Can you work these out from the model? Positions are in its coordinate system, mm. A direction names the side the tool comes from. Give positions to 0.01 mm unless a question says otherwise; leave off trailing zeros. Loops run counter-clockwise (first coordinate to the right, second up) from the corner with the lowest first, then second, coordinate; pieces in that order, holes last. Notation, with made-up numbers: (-3.75, 60) - (6.25, 60) arc R20 cw to (6.25, 99) - close; hole circle Ø11 at (49.5, -6.5). An arc over 180 degrees is marked (long way). Write item = value, one per line.
from build123d import *

# Parameters (mm, degrees)
BASE_DEPTH      = 10
ESQUISSE3_R     = 2.5
VIDE_TROU_DEPTH = 10
ESQUISSE4_R     = 4
AXE_DEPTH       = 90
CONG_5_R        = 1


with BuildPart() as part:
    # Esquisse2 → BASE (new body)
    with BuildSketch(Plane.XY):
        Polygon((-7.689490084, -15), (-2.689490084, -15), (-2.689490084, 0), (2.310509916, 0), (2.310509916, 9.990381057), (12.432116189, 27.521517376), (7.813314036, 27.521517376), (-2.689490084, 9.330127019), (-2.689490084, 15), (-7.689490084, 15), align=None)
    extrude(amount=BASE_DEPTH)

    # Esquisse3 → VIDE TROU (cut)
    with BuildSketch(Plane.ZY.offset(7.689490084)):
        with Locations((5, 5)):
            Circle(ESQUISSE3_R)
        with Locations((5, -5)):
            Circle(ESQUISSE3_R)
    extrude(amount=-VIDE_TROU_DEPTH, mode=Mode.SUBTRACT)

    # Esquisse4 → AXE (add)
    with BuildSketch(Plane(origin=(0, 27.521517376, 0), x_dir=(1, 0, 0), z_dir=(0, 1, 0))):
        with Locations(Location((10.122715113, -5, 0), (0, 0, 54.735610317))):
            Circle(ESQUISSE4_R)
    extrude(amount=AXE_DEPTH)

    # Congé5
    # the kernel refuses this fillet: 1 mm, written as the material it adds along each edge
    with BuildSketch(Plane(origin=(7.813314036, 27.521517376, -2.596113343), x_dir=(-0.500000000000004, -0.8660254037844363, 0), z_dir=(0, 0, 1))) as cong_5_piece_1_section:
        with BuildLine():
            CenterArc((CONG_5_R * 1.73205080757, -CONG_5_R), CONG_5_R, 90, 120)
            Line((CONG_5_R * 0.866025403784, -CONG_5_R * 1.5), (0, 0))
            Line((0, 0), (CONG_5_R * 1.73205080757, 0))
        make_face()
    cong_5_piece_1 = extrude(amount=15.192226685, mode=Mode.PRIVATE)
    cong_5_piece_1 = cong_5_piece_1 & Plane(origin=(10.122715113, 27.147514767, 5), x_dir=(0.577350269193122, 0, -0.8164965809252538), z_dir=(0, -1, 0)) * Cylinder(4, 38, mode=Mode.PRIVATE)
    add(cong_5_piece_1)
    with BuildSketch(Plane(origin=(12.432116189, 27.521517376, 0.290638003), x_dir=(-0.500000000000006, -0.8660254037844353, 0), z_dir=(0, 0, 1))) as cong_5_piece_2_section:
        with BuildLine():
            CenterArc((CONG_5_R * 0.57735026919, CONG_5_R), CONG_5_R, 210, 60)
            Line((-CONG_5_R * 0.288675134595, CONG_5_R * 0.5), (0, 0))
            Line((0, 0), (CONG_5_R * 0.57735026919, 0))
        make_face()
    cong_5_piece_2 = extrude(amount=9.418723993, mode=Mode.PRIVATE)
    cong_5_piece_2 = cong_5_piece_2 & Plane(origin=(10.122715113, 27.414246349, 5), x_dir=(0.577350269193122, 0, -0.8164965809252538), z_dir=(0, -1, 0)) * Cylinder(4, 22, mode=Mode.PRIVATE)
    add(cong_5_piece_2)


solid = part.part
Q1. Imagine slicing it at A-A, the plane y = -5. Write out the boundary of the cut face in (x, z).
Output:
outline = (-7.69, 0) - (-2.69, 0) - (-2.69, 2.5) - (-7.69, 2.5) - close; (-7.69, 7.5) - (-2.69, 7.5) - (-2.69, 10) - (-7.69, 10) - close
Q2. Imagine slicing it at C-C, the plane x = -5.25. Write out the boundary of the cut face in (y, z).
Output:
outline = (-15, 0) - (15, 0) - (15, 10) - (-15, 10) - close; hole circle Ø5 at (-5, 5); hole circle Ø5 at (5, 5)
Q3. Which directions (+Z, -Z, +X, -X, +Y, -Y) give clear straight access to the entire face, cutting with the end or side of a thin tool? Please do faces 1 (the flat face through (2.311, 3, 3)), 2 (the flat face through (-7.689, 0, 5)), 3 (the flat face through (-5, 15, 5)).
Output:
face_1 = +Z, -Z, +X, -Y
face_2 = +Z, -Z, -X, +Y, -Y
face_3 = +Z, -Z, -X, +Y
Q4. We'd pull the mould along Z, two halves only. Please class faces 4 (the flat face through (-5, -15, 5)), 5 (the flat face through (-1, 6, 0)), 6 (the cylindrical face through (-5.224, -4.249, 7.385)), 7 (the cylindrical face through (-2.759, 5.751, 7.385)): released by +Z, released by -Z, zero draft, split by the parting line, or undercut.
Output:
face_4 = zero draft
face_5 = released by -Z
face_6 = undercut
face_7 = undercut
Q5. I need wall thicknesses on L1, parallel to Y at x = -6.55, z = 5; L2, parallel to X at y = 90.5, z = 1.75; L3, parallel to Y at x = -6, z = 9.5. Which ranges of each line are inside material? Lowest first, please.
Output:
L1 = -15 to -7.5, -2.5 to 2.5, 7.5 to 15
L2 = 7.79 to 12.45
L3 = -15 to 15
Q6. For pin 1 (3 mm diameter, centred on y = 3.5, z = 5, fed in from +X); pin 2 (1.5 mm diameter, centred on x = 9, y = 32.5, fed in from -Z); pin 3 (5.5 mm diameter, centred on x = -4, z = 3, fed in from +Y); pin 4 (4 mm diameter, centred on x = 3, y = 32.5, fed in from -Z), each with a flat end and sliding along its axis, tell me the tip position at first contact or that it passes through.
Output:
pin_1 = 2.31
pin_2 = 1.02
pin_3 = 15
pin_4 = through
Q7. Imagine slicing it at D-D, the plane x = 9. Write out the boundary of the cut face in (y, z), then the cut area to 3 significant figures.
Output:
outline = (21.58, 0) - (27.52, 0) - (27.52, 1.16) - (117.52, 1.16) - (117.52, 8.84) - (27.52, 8.84) - (27.52, 10) - (21.58, 10) - close
area = 751 mm2
Q8. Imagine slicing it at B-B, the plane z = 3.75. Write out the boundary of the cut face in (x, y), then the cut area to 3 significant figures.
Output:
outline = (-7.69, -15) - (-2.69, -15) - (-2.69, -7.17) - (-7.69, -7.17) - close; (-7.69, -2.83) - (-2.69, -2.83) - (-2.69, 0) - (2.31, 0) - (2.31, 2.83) - (-7.69, 2.83) - close; (-7.69, 7.17) - (2.31, 7.17) - (2.31, 9.99) - (12.14, 27.02) arc R1 cw to (13.01, 27.52) - (13.92, 27.52) - (13.92, 117.52) - (6.32, 117.52) - (6.32, 27.49) arc R1 cw to (6.95, 26.02) - (-2.69, 9.33) - (-2.69, 15) - (-7.69, 15) - close
area = 901 mm2
